from build123d import *

# Parameters (mm, degrees)
F0_R     = 20.32
F1_DEPTH = 28.575
F2_R     = 6.35


with BuildPart() as f1:
    # F0 (on Top) → F1 (new body)
    with BuildSketch(Plane.XY):
        with BuildLine():
            ThreePointArc((23.9050999455, -6.4692674698), (24.5490837421, -3.2630832697), (24.765, 0))
            ThreePointArc((24.765, 0), (19.6285885254, 15.1004548773), (6.35, 23.9370575677))
            ThreePointArc((6.35, 23.9370575677), (4.0651088886, 24.4290833787), (1.7440091422, 24.703515076))
            ThreePointArc((1.7440091422, 24.703515076), (1.8643178935, 24.3286489263), (1.905, 23.9370575677))
            ThreePointArc((1.905, 23.9370575677), (-0.3915913586, 22.0727396742), (-1.7440091422, 24.703515076))
            ThreePointArc((-1.7440091422, 24.703515076), (-4.0651088886, 24.4290833787), (-6.35, 23.9370575677))
            ThreePointArc((-6.35, 23.9370575677), (-21.4471191247, 12.3825), (-23.9050999455, -6.4692674698))
            ThreePointArc((-23.9050999455, -6.4692674698), (-23.1887612414, -8.6940541227), (-22.2658761897, -10.8414013165))
            ThreePointArc((-22.2658761897, -10.8414013165), (-20.1370690632, -10.1581864481), (-18.8250999455, -11.9685287839))
            ThreePointArc((-18.8250999455, -11.9685287839), (-19.3113489683, -13.239815795), (-20.5218670475, -13.8621137596))
            ThreePointArc((-20.5218670475, -13.8621137596), (-19.1236523528, -15.735029256), (-17.5550999455, -17.4677900979))
            ThreePointArc((-17.5550999455, -17.4677900979), (0, -24.765), (17.5550999455, -17.4677900979))
            ThreePointArc((17.5550999455, -17.4677900979), (19.1236523528, -15.735029256), (20.5218670475, -13.8621137596))
            ThreePointArc((20.5218670475, -13.8621137596), (19.0803215513, -11.0160287839), (22.2658761897, -10.8414013165))
            ThreePointArc((22.2658761897, -10.8414013165), (23.1887612414, -8.6940541227), (23.9050999455, -6.4692674698))
        make_face()
        Circle(F0_R, mode=Mode.SUBTRACT)
        with BuildLine():
            ThreePointArc((-22.2658761897, -10.8414013165), (-23.1887612414, -8.6940541227), (-23.9050999455, -6.4692674698))
            ThreePointArc((-23.9050999455, -6.4692674698), (-26.2293612595, -15.1435287839), (-17.5550999455, -17.4677900979))
            ThreePointArc((-17.5550999455, -17.4677900979), (-19.1236523528, -15.735029256), (-20.5218670475, -13.8621137596))
            ThreePointArc((-20.5218670475, -13.8621137596), (-22.3798783397, -12.9210287839), (-22.2658761897, -10.8414013165))
        make_face()
        with BuildLine():
            ThreePointArc((1.7440091422, 24.703515076), (4.0651088886, 24.4290833787), (6.35, 23.9370575677))
            ThreePointArc((6.35, 23.9370575677), (0, 30.2870575677), (-6.35, 23.9370575677))
            ThreePointArc((-6.35, 23.9370575677), (-4.0651088886, 24.4290833787), (-1.7440091422, 24.703515076))
            ThreePointArc((-1.7440091422, 24.703515076), (0, 25.8420575677), (1.7440091422, 24.703515076))
        make_face()
        with BuildLine():
            ThreePointArc((17.5550999455, -17.4677900979), (26.2293612595, -15.1435287839), (23.9050999455, -6.4692674698))
            ThreePointArc((23.9050999455, -6.4692674698), (23.1887612414, -8.6940541227), (22.2658761897, -10.8414013165))
            ThreePointArc((22.2658761897, -10.8414013165), (22.5404422812, -11.3754979015), (22.6350999455, -11.9685287839))
            ThreePointArc((22.6350999455, -11.9685287839), (22.0013869566, -13.3872797611), (20.5218670475, -13.8621137596))
            ThreePointArc((20.5218670475, -13.8621137596), (19.1236523528, -15.735029256), (17.5550999455, -17.4677900979))
        make_face()
    extrude(amount=F1_DEPTH)

    # F2
    f2_edges = [f1.edges().sort_by_distance(p)[0] for p in [
        (6.35, 23.937058, 14.2875),
        (-23.9051, -6.469267, 14.2875),
        (17.5551, -17.46779, 14.2875),
        (23.9051, -6.469267, 14.2875),
        (-6.35, 23.937058, 14.2875),
        (-17.5551, -17.46779, 14.2875),
    ]]
    fillet(f2_edges, radius=F2_R)


solid = f1.part
For this review, take the finished solid that the model builds, in its own axes (mm). Coordinates: 2 decimals unless noted, no trailing zeros. Loops run counter-clockwise (first coordinate to the right, second up) from the corner with the lowest first, then second, coordinate; pieces in that order, holes last. Notation, with made-up numbers: (20, -7) -> (44, -7) arc R28 cw to (44, 19) -> close; hole circle Ø6 at (-30, 24). An arc over 180 degrees is marked (long way). Write each question's results on one line, items separated by ' | '.
Q1. Add section D-D, the plane x = -14. State the section outline as (y, z) points (3 decimals), then the cut area to 3 significant figures.
Taken from the geometry:
outline: (-20.428, 0) -> (-14.728, 0) -> (-14.728, 28.575) -> (-20.428, 28.575) -> close; (14.728, 0) -> (20.428, 0) -> (20.428, 28.575) -> (14.728, 28.575) -> close | area: 326 mm²
Q2. Add section A-A, the plane x = 0. State the section outline as (y, z) points (3 decimals).
Taken from the geometry:
outline: (-24.765, 0) -> (-20.32, 0) -> (-20.32, 28.575) -> (-24.765, 28.575) -> close; (20.32, 0) -> (22.032, 0) -> (22.032, 28.575) -> (20.32, 28.575) -> close; (25.842, 0) -> (30.287, 0) -> (30.287, 28.575) -> (25.842, 28.575) -> close
Q3. For pin 1 Ø6 at (x, z) = (21, 21.5) entering from +Y; pin 2 Ø6 at (x, y) = (0, 23.94) entering from -Z; pin 3 Ø12 at (x, z) = (4, 11) entering from -Y (3 decimals); pin 4 Ø1 at (y, z) = (4.5, 8) entering from +X, all flat-tipped, find the tip position at first contact; note any pin that passes through.
Taken from the geometry:
pin 1: y = 17.01 | pin 2: z = 0 | pin 3: y = -24.765 | pin 4: x = 24.44
Q4. To check wall thickness, follow line 1 along X through (y, z) = (3.5, 18); line 2 along X through (y, z) = (-8.5, 12.5); line 3 along Y through (x, z) = (-2, 26.25). State the ranges of each line that lie inside material, in increasing order. Write a range as [from, to].
Taken from the geometry:
line 1: [-24.52, -20.02], [20.02, 24.52] | line 2: [-26.05, -18.46], [18.46, 26.05] | line 3: [-24.68, -20.22], [20.22, 29.96]
Q5. Mouldability with a two-part tool opening along Y and no side actions: class faces 1 (the cylindrical face through (26.18, -15.23, 14.09)), 2 (the cylindrical face through (-2.645, 20.147, 14.087)), 3 (the cylindrical face through (0.105, 30.286, 14.087)), 4 (the flat face through (-14, 15, 28.575)) as +Y half, -Y half, draft (parallel to the pull), parting line (faces both ways), or undercut.
Taken from the geometry:
face 1: parting line | face 2: undercut | face 3: +Y half | face 4: draft
Q6. Add section B-B, the plane y = 15.5. State the section outline as (x, z) points (3 decimals).
Taken from the geometry:
outline: (-19.315, 0) -> (-13.14, 0) -> (-13.14, 28.575) -> (-19.315, 28.575) -> close; (13.14, 0) -> (19.315, 0) -> (19.315, 28.575) -> (13.14, 28.575) -> close
Q7. Add section C-C, the plane y = -13. State the section outline as (x, z) points (1 decimal).
Taken from the geometry:
outline: (-27, 0) -> (-22.3, 0) -> (-22.3, 28.6) -> (-27, 28.6) -> close; (-19.1, 0) -> (-15.6, 0) -> (-15.6, 28.6) -> (-19.1, 28.6) -> close; (15.6, 0) -> (19.1, 0) -> (19.1, 28.6) -> (15.6, 28.6) -> close; (22.3, 0) -> (27, 0) -> (27, 28.6) -> (22.3, 28.6) -> close
